Source: CAD feature listing. Evaluate the final solid. Frame: model axes, mm. Coordinates: 2 decimals unless noted, no trailing zeros. Write each loop counter-clockwise with the first axis right and the second up, starting at its lowest first coordinate (ties: lowest second). Pieces come first, ordered by that corner, then holes. Notation, with made-up numbers: M 64,-28 L 88,-28 A17 ccw 88,3 Z; hole C 36,47.25 d5. An arc over 180 degrees is marked long. One line per item, written item: value. Start each with the question number.
Item 1: Cut plane C-C, the plane y = 3. Output: boundary loops of the cut face in (x, z).
Item 2: Cut plane B-B, the plane y = 27. Output: boundary loops of the cut face in (x, z), then the cut area to 3 significant figures.
Item 3: Ray query, L1, parallel to X at y = 7.5, z = 0; L2, parallel to Z at x = 3.5, y = 7. Return the intervals inside material, ascending. Write a range as from..to.
Item 4: Cut plane A-A, the plane z = 0. Output: boundary loops of the cut face in (x, y).
Item 5: Pin query (flat end, axial travel): P1, Ø7.5, axis at x = 0, z = 0, coming from the -Y side; P2, Ø8, axis at y = 10.5, z = -4.5, coming from the -X side; P3, Ø1.5, axis at x = -2.5, y = 5, coming from the +Z side; P4, Ø4, axis at y = 4, z = 3.5, coming from the +X side. Return the tip coordinate at first contact, or that it passes through.
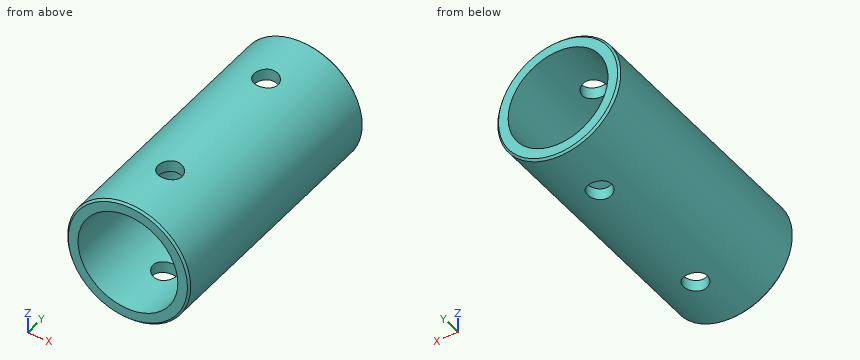
```python
from build123d import *

# Parameters (mm, degrees)
SKETCH1_R               = 7.94
SKETCH1_R_2             = 6.44
BOSS_EXTRUDE1_DEPTH     = 33.7
CHAMFER1_SIZE           = 0.25
SKETCH2_R               = 1.55
SKETCH2_RX              = 1.55
SKETCH2_RY              = 1.54981566
CUT_EXTRUDE1_DEPTH      = 3.443979861
CUT_EXTRUDE1_DEPTH_BACK = 15.143979861


with BuildPart() as part:
    # Sketch1 → Boss-Extrude1 (new body)
    with BuildSketch(Plane(origin=(0, 0, 0), x_dir=(1, 0, 0), z_dir=(0, 1, 0))):
        Circle(SKETCH1_R)
        Circle(SKETCH1_R_2, mode=Mode.SUBTRACT)
    extrude(amount=BOSS_EXTRUDE1_DEPTH)

    # Chamfer1
    chamfer1_edges = [part.edges().sort_by_distance(p)[0] for p in [
        (-7.94, 0, 0),
        (-7.94, 33.7, 0),
    ]]
    chamfer(chamfer1_edges, length=CHAMFER1_SIZE)

    # Sketch2 → Cut-Extrude1 (cut, two sides)
    with BuildSketch(Plane(origin=(0.266895271, 0, 5.843908531), x_dir=(0.998958723, 0, -0.045623123), z_dir=(0.045623123, 0, 0.998958723))) as cut_extrude1_sk:
        with Locations((0, 26.2)):
            Circle(SKETCH2_R)
        with Locations(Location((0.090219685, 7.5), (0, 0, 90))):
            Ellipse(SKETCH2_RX, SKETCH2_RY)
    extrude(amount=CUT_EXTRUDE1_DEPTH, mode=Mode.SUBTRACT)
    extrude(cut_extrude1_sk.sketch, amount=-CUT_EXTRUDE1_DEPTH_BACK, mode=Mode.SUBTRACT)


solid = part.part
```
From the geometry:
1. outline: C 0,0 d15.88; hole C 0,0 d12.88
2. outline: M -1.68,-7.76 L -1.61,-6.23 A6.44 cw -1.04,6.36 L -0.97,7.88 A7.94 ccw Z; M 0.97,-7.88 A7.94 ccw 1.68,7.76 L 1.61,6.23 A6.44 cw 1.04,-6.36 Z
2. area: 59.8 mm²
3. L1: x = -7.94..-6.44, 6.44..7.94
3. L2: z = -7.13..-5.41, 5.41..7.13
4. outline: M -7.94,0.25 L -7.69,0 L -6.44,0 L -6.44,33.7 L -7.69,33.7 L -7.94,33.45 Z; M 6.44,0 L 7.69,0 L 7.94,0.25 L 7.94,33.45 L 7.69,33.7 L 6.44,33.7 Z
5. P1: passes through
5. P2: stops at x = -7.92
5. P3: stops at z = 7.74
5. P4: stops at x = 7.8
